```python
from build123d import *

# Parameters (mm, degrees)
SKETCH_W        = 90
SKETCH_H        = 60
SKETCH_R        = 3.25
PAD_DEPTH       = 11
SKETCH001_R     = 6.1
POCKET_DEPTH    = 4
POCKET001_DEPTH = 5.25
FILLET_R        = 4
CHAMFER_SIZE    = 0.4
CHAMFER001_SIZE = 0.4


with BuildPart() as part:
    # Sketch → Pad (new body)
    with BuildSketch(Plane.XY):
        with Locations((45, 30)):
            Rectangle(SKETCH_W, SKETCH_H)
        with Locations((10, 40)):
            Circle(SKETCH_R, mode=Mode.SUBTRACT)
        with Locations((80, 40)):
            Circle(SKETCH_R, mode=Mode.SUBTRACT)
        with Locations((10, 20)):
            Circle(SKETCH_R, mode=Mode.SUBTRACT)
        with Locations((80, 20)):
            Circle(SKETCH_R, mode=Mode.SUBTRACT)
        with Locations((15, 50)):
            Circle(SKETCH_R, mode=Mode.SUBTRACT)
        with Locations((75, 50)):
            Circle(SKETCH_R, mode=Mode.SUBTRACT)
        with Locations((75, 10)):
            Circle(SKETCH_R, mode=Mode.SUBTRACT)
        with Locations((15, 10)):
            Circle(SKETCH_R, mode=Mode.SUBTRACT)
    extrude(amount=PAD_DEPTH)

    # Sketch001 (on Face14 of Pad) → Pocket (cut)
    with BuildSketch(Plane.XY.offset(11)):
        with Locations((15, 50)):
            Circle(SKETCH001_R)
        with Locations((75, 50)):
            Circle(SKETCH001_R)
        with Locations((75, 10)):
            Circle(SKETCH001_R)
        with Locations((15, 10)):
            Circle(SKETCH001_R)
    extrude(amount=-POCKET_DEPTH, mode=Mode.SUBTRACT)

    # Sketch002 (on Face4 of Pocket) → Pocket001 (cut)
    with BuildSketch(Plane(origin=(0, 0, 0), x_dir=(1, 0, 0), z_dir=(0, 0, -1))):
        Polygon((15.1, -17.055514), (10, -14.111027), (4.9, -17.055514), (4.9, -22.944486), (10, -25.888973), (15.1, -22.944486), align=None)
        Polygon((80, -14.111027), (74.9, -17.055514), (74.9, -22.944486), (80, -25.888973), (85.1, -22.944486), (85.1, -17.055514), align=None)
        Polygon((10, -34.111027), (4.9, -37.055514), (4.9, -42.944486), (10, -45.888973), (15.1, -42.944486), (15.1, -37.055514), align=None)
        Polygon((80, -34.111027), (74.9, -37.055514), (74.9, -42.944486), (80, -45.888973), (85.1, -42.944486), (85.1, -37.055514), align=None)
    extrude(amount=-POCKET001_DEPTH, mode=Mode.SUBTRACT)

    # Fillet
    fillet_edges = [part.edges().sort_by_distance(p)[0] for p in [
        (0, 60, 5.5),
        (90, 60, 5.5),
        (90, 0, 5.5),
        (0, 0, 5.5),
    ]]
    fillet(fillet_edges, radius=FILLET_R)

    # Chamfer
    chamfer_edges = [part.edges().sort_by_distance(p)[0] for p in [
        (45, 60, 11),
        (1.171573, 58.828427, 11),
        (88.828427, 58.828427, 11),
        (0, 30, 11),
        (90, 30, 11),
        (1.171573, 1.171573, 11),
        (88.828427, 1.171573, 11),
        (45, 0, 11),
        (68.9, 10, 11),
        (76.75, 20, 11),
        (8.9, 10, 11),
        (6.75, 20, 11),
        (76.75, 40, 11),
        (68.9, 50, 11),
        (6.75, 40, 11),
        (8.9, 50, 11),
    ]]
    chamfer(chamfer_edges, length=CHAMFER_SIZE)

    # Chamfer001
    chamfer001_edges = [part.edges().sort_by_distance(p)[0] for p in [
        (45, 60, 0),
        (1.171573, 58.828427, 0),
        (88.828427, 58.828427, 0),
        (0, 30, 0),
        (90, 30, 0),
        (1.171573, 1.171573, 0),
        (88.828427, 1.171573, 0),
        (45, 0, 0),
        (71.75, 10, 0),
        (77.45, 15.58327, 0),
        (74.9, 20, 0),
        (77.45, 24.41673, 0),
        (82.55, 24.41673, 0),
        (85.1, 20, 0),
        (82.55, 15.58327, 0),
        (11.75, 10, 0),
        (12.55, 15.58327, 0),
        (7.45, 15.58327, 0),
        (4.9, 20, 0),
        (7.45, 24.41673, 0),
        (12.55, 24.41673, 0),
        (15.1, 20, 0),
        (77.45, 35.58327, 0),
        (74.9, 40, 0),
        (77.45, 44.41673, 0),
        (82.55, 44.41673, 0),
        (85.1, 40, 0),
        (82.55, 35.58327, 0),
        (71.75, 50, 0),
        (7.45, 35.58327, 0),
        (4.9, 40, 0),
        (7.45, 44.41673, 0),
        (12.55, 44.41673, 0),
        (15.1, 40, 0),
        (12.55, 35.58327, 0),
        (11.75, 50, 0),
    ]]
    chamfer(chamfer001_edges, length=CHAMFER001_SIZE)


solid = part.part
```
Source: CAD feature listing. Evaluate the final solid. Frame: model axes, mm. A direction names the side the tool comes from. Round coordinates to 2 decimals unless told otherwise and drop trailing zeros. Use a Markdown table: item, result. Add a question column.
1. Pull-direction query (X, two-part tool) for faces 1 (the flat face through (0, 30, 5)), 2 (the flat face through (18, 7, 7)), 3 (the conical face through (88.65, 1.4, 0.11)), 4 (the flat face through (77.49, 35.56, 2.79)); classes: +X half, -X half, draft (parallel to the pull), parting line (faces both ways), or undercut.
2. Cut plane A-A, the plane y = 10. State how many separate pieces and enclosed holes the cut face has, and give its area (3 significant figures).
3. Ray query, line 1 along Y through (x, z) = (15, 5.5); line 2 along Y through (x, z) = (15, 7.8); line 3 along X through (y, z) = (20, 8). Return the intervals inside material, ascending. Write a range as [from, to].
4. Contact query for flat-ended pins moving along their axis: pin 1 (10 mm diameter, centred on x = 15, y = 50, fed in from +Z); pin 2 (3 mm diameter, centred on x = 81.5, y = 22, fed in from -Z); pin 3 (10.5 mm diameter, centred on x = 80, y = 20, fed in from -Z); pin 4 (4 mm diameter, centred on x = 15, y = 10, fed in from -Z). Output: stop coordinate, or through.
5. Set-up query: faces 5 (the cylindrical face through (14.295, 46.827, 3.654)), 6 (the flat face through (77.49, 15.56, 2.79)), 7 (the cylindrical face through (13.678, 4.045, 8.825)). Return all of +Z, -Z, +X, -X, +Y, -Y with unobstructed straight access to the full face (end or side cutting, diameter ignored); none if empty.
Solution:
| question | item | result |
|---|---|---|
| 1 | face 1 | -X half |
| 1 | face 2 | undercut |
| 1 | face 3 | +X half |
| 1 | face 4 | undercut |
| 2 | separate pieces | 3 |
| 2 | enclosed holes | 0 |
| 2 | area | 800 mm2 |
| 3 | line 1 | y = [0, 6.75], [13.25, 46.75], [53.25, 60] |
| 3 | line 2 | y = [0, 3.9], [16.1, 43.9], [56.1, 60] |
| 3 | line 3 | x = [0, 6.75], [13.25, 76.75], [83.25, 90] |
| 4 | pin 1 | stops at z = 7 |
| 4 | pin 2 | stops at z = 5.25 |
| 4 | pin 3 | stops at z = 0.25 |
| 4 | pin 4 | passes through |
| 5 | face 5 | +Z, -Z |
| 5 | face 6 | -Z |
| 5 | face 7 | +Z |
